```python
from build123d import *

# Parameters (mm, degrees)
SKETCH1_W = 25
SKETCH1_H = 25


with BuildPart() as part:
    # Sketch1 → Revolve1 (revolve)
    with BuildSketch(Plane.XY, mode=Mode.PRIVATE) as revolve1_sk:
        Polygon((-230.074626866, 25), (-330.074626866, 25), (-330.074626866, 0), (349.925373134, 0), (349.925373134, 50), (319.925373134, 50), (319.925373134, 25), (219.925373134, 25), (219.925373134, 55), (-230.074626866, 55), align=None)
        with Locations((362.425373134, 12.5)):
            Rectangle(SKETCH1_W, SKETCH1_H)
    revolve(revolve1_sk.sketch.rotate(Axis((-330.074626866, 0, 0), (1, 0, 0)), 180), axis=Axis((-330.074626866, 0, 0), (1, 0, 0)))


solid = part.part
```
Work out the finished part from the listing and answer in its coordinate system (mm). A direction names the side the tool comes from. Round coordinates to 2 decimals unless told otherwise and drop trailing zeros. Order: outer loops, then holes, each group sorted by start corner. A loop starts at its lowest first (then second) coordinate and runs counter-clockwise, first axis right, second up.
Q1. A tool of negligible diameter and unlimited length cuts with its end or side. For faces 4 (the cylindrical face through (362.6, -23.846, -7.509)), 5 (the flat face through (219.925, 24, 11)), 6 (the flat face through (-230.075, -11, 24)), from which of +Z, -Z, +X, -X, +Y, -Y can it reach the whole face along a straight path? Write none if from no direction.
Solution:
face 4: +X
face 5: none
face 6: -X
Q2. A cutting plane is placed at D-D, the plane x = -2.5. Determine the outline of the cut face in (y, z).
Solution:
outline: circle Ø110 at (0, 0)
Q3. Given pin 1 Ø2 at (x, z) = (159.5, -42.5) entering from +Y; pin 2 Ø8 at (x, z) = (292.5, 19) entering from -Y; pin 3 Ø12 at (x, z) = (-134.5, 12.5) entering from -Y, each flat-ended and moving along its own axis, determine where each tip first touches the part or whether it passes through.
Solution:
pin 1: stops at y = 36.09
pin 2: stops at y = -20
pin 3: stops at y = -54.61
Q4. A cutting plane is placed at A-A, the plane z = -41. Determine the outline of the cut face in (x, y).
Solution:
outline: (-230.07, -36.66) - (219.93, -36.66) - (219.93, 36.66) - (-230.07, 36.66) - close; (319.93, -28.62) - (349.93, -28.62) - (349.93, 28.62) - (319.93, 28.62) - close
Q5. A cutting plane is placed at B-B, the plane y = 0. Determine the outline of the cut face in (x, z).
Solution:
outline: (-330.07, -25) - (-230.07, -25) - (-230.07, -55) - (219.93, -55) - (219.93, -25) - (319.93, -25) - (319.93, -50) - (349.93, -50) - (349.93, -25) - (374.93, -25) - (374.93, 25) - (349.93, 25) - (349.93, 50) - (319.93, 50) - (319.93, 25) - (219.93, 25) - (219.93, 55) - (-230.07, 55) - (-230.07, 25) - (-330.07, 25) - close
Q6. The mould has two halves that part along X. Classify faces 1 (the cylindrical face through (-280.775, -23.846, -7.509)), 2 (the flat face through (319.925, 22.9, 10.4)), 3 (the flat face through (349.925, 10.4, -22.9)): pulls with the +X half, pulls with the -X half, needs draft (parallel to the pull), parting line crosses it, or undercut.
Solution:
face 1: needs draft
face 2: undercut
face 3: pulls with the +X half
Q7. Find the intervals of material crossed by line 1 along X through (y, z) = (-6, 25.5); line 2 along X through (y, z) = (-25.5, -48); line 3 along Z through (x, y) = (163.5, 3), in increasing order.
Solution:
line 1: x = -230.07 to 219.93, 319.93 to 349.93
line 2: x = -230.07 to 219.93
line 3: z = -54.92 to 54.92
